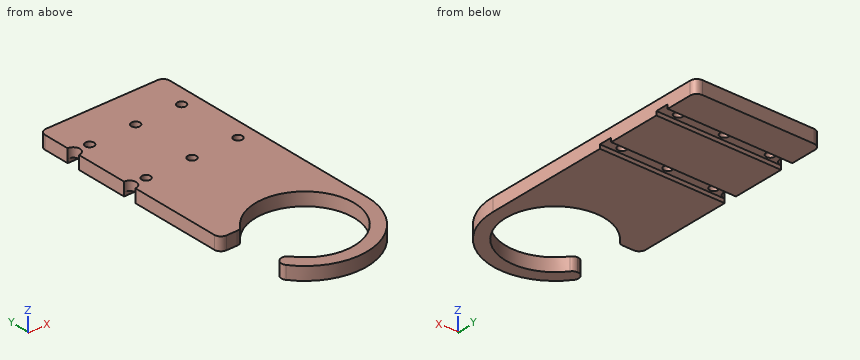
from build123d import *

# Parameters (mm, degrees)
SKETCH_1_R          = 3.3
EXTRUDE_1_DEPTH     = 10
SKETCH_1_4_R        = 3.3
CUT_EXTRUDE_1_DEPTH = 3
FILLET_4_R          = 5
FILLET_8_R          = 5


with BuildPart() as part:
    # 스케치1 → 보스-돌출1 (new body)
    with BuildSketch(Plane.XY):
        with BuildLine():
            Line((-47.5, 95), (-47.5, 20))
            Line((-47.5, 20), (-31.721443851, 20))
            ThreePointArc((-31.721443851, 20), (37.5, 0), (-31.721443851, -20))
            Line((-31.721443851, -20), (-43.084219849, -20))
            ThreePointArc((-43.084219849, -20), (10.240838764, -46.382919501), (47.5, 0))
            Line((47.5, 0), (47.5, 180))
            Line((47.5, 180), (-47.5, 180))
            Line((-47.5, 180), (-47.5, 155))
            ThreePointArc((-47.5, 155), (-42.5, 150), (-47.5, 145))
            Line((-47.5, 145), (-47.5, 105))
            ThreePointArc((-47.5, 105), (-42.5, 100), (-47.5, 95))
        make_face()
        with Locations((35, 100)):
            Circle(SKETCH_1_R, mode=Mode.SUBTRACT)
        with Locations((-35, 100)):
            Circle(SKETCH_1_R, mode=Mode.SUBTRACT)
        with Locations((0, 100)):
            Circle(SKETCH_1_R, mode=Mode.SUBTRACT)
        with Locations((35, 150)):
            Circle(SKETCH_1_R, mode=Mode.SUBTRACT)
        with Locations((-35, 150)):
            Circle(SKETCH_1_R, mode=Mode.SUBTRACT)
        with Locations((0, 150)):
            Circle(SKETCH_1_R, mode=Mode.SUBTRACT)
    extrude(amount=EXTRUDE_1_DEPTH)

    # 스케치1<4> → 컷-돌출1 (cut)
    # profile 1 of 2: a face of its own
    with BuildSketch(Plane.XY):
        with BuildLine():
            ThreePointArc((-47.5, 105), (-42.5, 100), (-47.5, 95))
            Line((-47.5, 95), (47.5, 95))
            Line((47.5, 95), (47.5, 105))
            Line((47.5, 105), (-47.5, 105))
        make_face()
        with Locations((-35, 100)):
            Circle(SKETCH_1_4_R, mode=Mode.SUBTRACT)
        with Locations((0, 100)):
            Circle(SKETCH_1_4_R, mode=Mode.SUBTRACT)
        with Locations((35, 100)):
            Circle(SKETCH_1_4_R, mode=Mode.SUBTRACT)
    # profile 2 of 2: a face of its own
    with BuildSketch(Plane.XY):
        with BuildLine():
            ThreePointArc((-47.5, 155), (-42.5, 150), (-47.5, 145))
            Line((-47.5, 145), (47.5, 145))
            Line((47.5, 145), (47.5, 155))
            Line((47.5, 155), (-47.5, 155))
        make_face()
        with Locations((-35, 150)):
            Circle(SKETCH_1_4_R, mode=Mode.SUBTRACT)
        with Locations((0, 150)):
            Circle(SKETCH_1_4_R, mode=Mode.SUBTRACT)
        with Locations((35, 150)):
            Circle(SKETCH_1_4_R, mode=Mode.SUBTRACT)
    extrude(amount=CUT_EXTRUDE_1_DEPTH, mode=Mode.SUBTRACT)

    # 필렛4
    fillet_4_edges = [part.edges().sort_by_distance(p)[0] for p in [
        (-31.721443851, 20, 5),
        (-47.5, 20, 5),
        (-31.721443851, -20, 5),
        (-43.084219849, -20, 5),
    ]]
    fillet(fillet_4_edges, radius=FILLET_4_R - 0.0001)  # a hair under: the kernel refuses the full size

    # 필렛8
    fillet_8_edges = [part.edges().sort_by_distance(p)[0] for p in [
        (-47.5, 180, 5),
        (47.5, 180, 5),
    ]]
    fillet(fillet_8_edges, radius=FILLET_8_R)


solid = part.part
Here's how the part is built. I have some questions about the finished solid (model axes, mm). Coordinates: 2 decimals unless noted, no trailing zeros. Order: outer loops, then holes, each group sorted by start corner. A loop starts at its lowest first (then second) coordinate and runs counter-clockwise, first axis right, second up. Notation, with made-up numbers: (18.25, -0.75) - (46.25, -0.75) arc R25 ccw to (46.25, 26.25) - close; hole circle Ø2 at (0, -39). An arc over 180 degrees is marked (long way). Use CSV: the item, a comma, the result in double quotes. Start each with the question number.
1. Suppose I cut it at D-D on x = 0.5. List the corners of the cut face in (y, z) for me, then the cut area to 3 significant figures.
2. I'm going to push flat-ended pins straight in: pin 1 (0.9 mm diameter, centred on x = 7.5, z = 2, fed in from -Y); pin 2 (7.5 mm diameter, centred on x = -35, y = 150, fed in from -Z); pin 3 (1 mm diameter, centred on y = 13, z = 1.5, fed in from -X). Where does each tip first touch, or does it pass through?
3. Suppose I cut it at A-A on z = 1.5. Give the number of separate pieces and of enclosed holes in the cut face, then the cut area to 3 significant figures.
4. Suppose I cut it at B-B on x = 14. List the corners of the cut face in (y, z) for me, then the cut area to 3 significant figures.
5. Suppose I cut it at C-C on y = 150. List the corners of the cut face in (x, z) for me.
6. Please list where these lines run through material, in increasing order: line 1 (Y direction, x = -35, z = 7.75); line 2 (Y direction, x = -12, z = 2.5); line 3 (Z direction, x = 16.5, y = 103.5). Write a range as from..to.
Output:
1,outline,"(-47.5, 0) - (-37.5, 0) - (-37.5, 10) - (-47.5, 10) - close; (37.5, 0) - (95, 0) - (95, 3) - (96.74, 3) - (96.74, 10) - (37.5, 10) - close; (103.26, 3) - (105, 3) - (105, 0) - (145, 0) - (145, 3) - (146.74, 3) - (146.74, 10) - (103.26, 10) - close; (153.26, 3) - (155, 3) - (155, 0) - (180, 0) - (180, 10) - (153.26, 10) - close"
1,area,"1,370 mm2"
2,pin 1,"stops at y = -46.97"
2,pin 2,"stops at z = 3"
2,pin 3,"stops at x = 34.99"
3,separate pieces,"3"
3,enclosed holes,"0"
3,area,"13,800 mm2"
4,outline,"(-45.39, 0) - (-34.79, 0) - (-34.79, 10) - (-45.39, 10) - close; (34.79, 0) - (95, 0) - (95, 3) - (105, 3) - (105, 0) - (145, 0) - (145, 3) - (155, 3) - (155, 0) - (180, 0) - (180, 10) - (34.79, 10) - close"
4,area,"1,500 mm2"
5,outline,"(-42.5, 3) - (-38.3, 3) - (-38.3, 10) - (-42.5, 10) - close; (-31.7, 3) - (-3.3, 3) - (-3.3, 10) - (-31.7, 10) - close; (3.3, 3) - (31.7, 3) - (31.7, 10) - (3.3, 10) - close; (38.3, 3) - (47.5, 3) - (47.5, 10) - (38.3, 10) - close"
6,line 1,"y = -32.11..-20.04, 20..96.7, 103.3..146.7, 153.3..180"
6,line 2,"y = -45.96..-35.53, 35.53..95, 105..145, 155..180"
6,line 3,"z = 3..10"
